Geometry check sheet. Reference: the model listing, model coordinates, mm. Give positions to 0.01 mm unless a question says otherwise; leave off trailing zeros. Write each loop counter-clockwise with the first axis right and the second up, starting at its lowest first coordinate (ties: lowest second). Pieces come first, ordered by that corner, then holes. Notation, with made-up numbers: (-3, 5.5) -> (11, 5.5) arc R24 cw to (11, 34.5) -> close; hole circle Ø1 at (-10.75, -9.5). An arc over 180 degrees is marked (long way). One line per item, written item: value.
from build123d import *

# Parameters (mm, degrees)
UP_DEPTH = 1.6


with BuildPart() as part:
    # Sketch1 → Up (new body)
    with BuildSketch(Plane(origin=(0, 0, 0), x_dir=(0, 0, -1), z_dir=(1, 0, 0))):
        Polygon((-216.6666645, 23.75), (-177.4327255, 23.75), (-177.4327255, 25.51), (-137.7187865, 25.51), (-137.7187865, 23.75), (-98.6448475, 23.75), (-98.6448475, 25.51), (-58.9309085, 25.51), (-58.9309085, 23.75), (-19.8569695, 23.75), (-19.8569695, 25.51), (19.8569695, 25.51), (19.8569695, 23.75), (58.9309085, 23.75), (58.9309085, 25.51), (98.6448475, 25.51), (98.6448475, 23.75), (137.7187865, 23.75), (137.7187865, 25.51), (177.4327255, 25.51), (177.4327255, 23.75), (216.6666645, 23.75), (218.4266645, 23.75), (218.4266645, 7.916666667), (216.6666645, 7.916666667), (216.6666645, 0), (-216.6666645, 0), (-218.4266645, 0), (-218.4266645, 7.916666667), (-216.6666645, 7.916666667), align=None)
    up = extrude(amount=UP_DEPTH)

    # Mirror2: Up across plane
    add(up.mirror(Plane(origin=(1.6, 0, 216.6666645), x_dir=(0, 0, 1), z_dir=(0, 1, 0))))


solid = part.part
1) Depth check by flat-ended pin: pin 1 Ø0.8 at (x, y) = (0.5, -25) entering from -Z; pin 2 Ø0.5 at (x, z) = (1, 32) entering from -Y. Enter the tip coordinate at first touch or a pass-through.
Verdict:
pin 1: z = -177.43
pin 2: y = -23.75
2) Scan lines: probe 1 along Z at (x, y) = (0.6, 10); probe 2 along Y at (x, z) = (0.75, 177.5); probe 3 along Z at (x, y) = (0.25, -5). Record each from-to range of solid material in increasing order.
Verdict:
probe 1: -218.43 to 216.67
probe 2: -23.75 to 23.75
probe 3: -216.67 to 218.43
3) Sectioned sample at A-A on z = 26. Record the cut outline in (x, y).
Verdict:
outline: (0, -23.75) -> (1.6, -23.75) -> (1.6, 23.75) -> (0, 23.75) -> close
